```python
from build123d import *
from build123d import SkipClean  # not in build123d's __all__

# Parameters (mm, degrees)
F0_W     = 12.7
F0_H     = 6.9
F1_DEPTH = 8.9
F3_DEPTH = 5
F8_W     = 0.76
F8_H     = 2.5
F9_DEPTH = 3.9


with BuildPart() as f1:
    # F0 (on Top) → F1 (new body)
    with BuildSketch(Plane.XY):
        with Locations((6.35, 0)):
            Rectangle(F0_W, F0_H)
    extrude(amount=F1_DEPTH)

    # F2 (on face) → F3 (join)
    with BuildSketch(Plane.XY.offset(8.9)):
        with BuildLine():
            ThreePointArc((6.35, -3.45), (8.7895183951, -2.4395183951), (9.8, 0))
            ThreePointArc((9.8, 0), (8.7895183951, 2.4395183951), (6.35, 3.45))
            ThreePointArc((6.35, 3.45), (2.9, 0), (6.35, -3.45))
        make_face()
    extrude(amount=F3_DEPTH)

    # F4 (on Front) → F5 (revolve)
    with BuildSketch(Plane.XZ):
        with BuildLine():
            Line((0.9029362769, 21.0829250706), (5.05, 13.9))
            Line((5.05, 13.9), (6.35, 13.9))
            Line((6.35, 13.9), (1.4796313262, 23.0890972887))
            ThreePointArc((1.4796313262, 23.0890972887), (0.7651079647, 22.2085198521), (0.9029362769, 21.0829250706))
        make_face()
    revolve(axis=Axis((3.9148156631, 0, 18.4945486443), (0.4683046802, 0, -0.883567047)))

    # F6 (on Front) → F7 (revolve)
    with BuildSketch(Plane.XZ):
        with BuildLine():
            ThreePointArc((8.35, 13.9), (6.35, 15.9), (4.35, 13.9))
            Line((4.35, 13.9), (8.35, 13.9))
        make_face()
    with SkipClean():  # cleaning this boolean's faces spoils the solid; the shape is the same uncleaned
        revolve(axis=Axis((6.35, 0, 13.9), (1, 0, 0)))

    # F8 (on Top) → F9 (join)
    with BuildSketch(Plane.XY):
        with Locations((1.65, 0)):
            Rectangle(F8_W, F8_H)
        with Locations((6.35, 0)):
            Rectangle(F8_W, F8_H)
        with Locations((11.05, 0)):
            Rectangle(F8_W, F8_H)
    with SkipClean():  # cleaning this boolean's faces spoils the solid; the shape is the same uncleaned
        extrude(amount=-F9_DEPTH)


solid = f1.part
```
Check sheet for the modelled part. Datum: model origin and axes. Units: mm. A direction names the side the tool comes from. Round coordinates to 2 decimals unless told otherwise and drop trailing zeros. Order: outer loops, then holes, each group sorted by start corner. A loop starts at its lowest first (then second) coordinate and runs counter-clockwise, first axis right, second up. Notation, with made-up numbers: (87.25, 41.25) -> (137.25, 41.25) arc R24 cw to (137.25, 79.25) -> close; hole circle Ø5 at (63.25, 28). An arc over 180 degrees is marked (long way). One line per item, written item: value. Start each with the question number.
Q1. Gauge pin test, flat ends, axial feed: pin 1 Ø1 at (y, z) = (-0.5, 19) entering from -X; pin 2 Ø0.6 at (x, z) = (6.5, -1.5) entering from -Y; pin 3 Ø2 at (x, z) = (7, -0.5) entering from +Y; pin 4 Ø0.6 at (x, z) = (1.5, -3) entering from +Y. Record the tip position at first contact, or that the pin passes through.
Q2. Cross-section at A-A (z = 10.5). Record the boundary of the cut face in (x, y).
Q3. Thickness scan on line 1 (Z direction, x = 8.5, y = -3); line 2 (Z direction, x = 9, y = 1); line 3 (Z direction, x = 1.5, y = 0). Record the ranges inside material, lowest first.
Q4. Set-up check for faces 4 (the face through (6.73, 0, -2)), 5 (the face through (6.3, -2.3, 13.9)), 6 (the face through (1.27, 0, -2)): record each of +Z, -Z, +X, -X, +Y, -Y from which the full face is reachable in a straight line by a thin tool's end or side.
Q5. Mould release check, pull along Z, two halves, no side actions. Record for faces 1 (the face through (2, 0, 8.9)), 2 (the face through (11, 0, 8.9)), 3 (the face through (6, 3.45, 4)): pulls with the +Z half, pulls with the -Z half, needs draft (parallel to the pull), parting line crosses it, or undercut.
Q6. Cross-section at C-C (y = 2.5). Record the boundary of the cut face in (x, z).
Q7. Cross-section at B-B (x = 8). Record the boundary of the cut face in (y, z).
Completed:
1. pin 1: stops at x = 1.88
1. pin 2: stops at y = -1.25
1. pin 3: stops at y = 3.45
1. pin 4: stops at y = 1.25
2. outline: circle Ø6.9 at (6.35, 0)
3. line 1: z = 0 to 8.9
3. line 2: z = 0 to 13.9
3. line 3: z = -3.9 to 8.9, 20.05 to 23.1
4. face 4: -Z, +Y, -Y
4. face 5: none
4. face 6: -Z, -X, +Y, -Y
5. face 1: undercut
5. face 2: pulls with the +Z half
5. face 3: needs draft
6. outline: (0, 0) -> (12.7, 0) -> (12.7, 8.9) -> (8.73, 8.9) -> (8.73, 13.9) -> (3.97, 13.9) -> (3.97, 8.9) -> (0, 8.9) -> close
7. outline: (-3.45, 0) -> (3.45, 0) -> (3.45, 8.9) -> (3.03, 8.9) -> (3.03, 13.9) -> (1.13, 13.9) arc R1.13 ccw to (-1.13, 13.9) -> (-3.03, 13.9) -> (-3.03, 8.9) -> (-3.45, 8.9) -> close
